```python
from build123d import *

# Parameters (mm, degrees)
F0_W     = 73
F0_H     = 125
F1_DEPTH = 5
F2_D     = 2.5
F3_D     = 3.3
F4_R     = 5
F7_DEPTH = 25
F8_D     = 2.5


# Not quite as in the source:
# - a feature names something its author has since deleted; it is built from what else it names


with BuildPart() as f1:
    # F0 (on Top) → F1 (new body)
    with BuildSketch(Plane.XY):
        with Locations((-1.7126457989, 19.3158909678)):
            Rectangle(F0_W, F0_H)
    extrude(amount=F1_DEPTH)

    # F2 (through all)
    with Locations(Plane(origin=(0, 0, 0), x_dir=(1, 0, 0), z_dir=(0, 0, -1))):
        with Locations((-30.3091388196, -76.7177641392), (27.6908611804, -76.7177641392), (27.6908611804, -53.7177641392), (-30.3091388196, -53.7177641392)):
            Hole(F2_D / 2)

    # F3 (through all)
    with Locations(Plane(origin=(0, 0, 0), x_dir=(1, 0, 0), z_dir=(0, 0, -1))):
        with Locations((-21.0855398327, -47.0293052495), (-13.0855398327, -47.0293052495)):
            Hole(F3_D / 2)

    # F4
    f4_edges = [f1.edges().sort_by_distance(p)[0] for p in [
        (-38.212646, 81.815891, 2.5),
        (34.787354, 81.815891, 2.5),
        (34.787354, -43.184109, 2.5),
        (-38.212646, -43.184109, 2.5),
    ]]
    fillet(f4_edges, radius=F4_R)

    # F5 (on face) → F7 (cut)
    with BuildSketch(Plane.XY.offset(5)):
        Polygon((19.4577450805, 31.105422746), (2.7185706181, 48.1802586667), (-26.0799791984, 20.3202102417), (-26.0799791984, -12.9482956412), align=None)
        Polygon((29.5474557331, 26.9350063375), (-26.0799791984, -26.8796142191), (29.5474557331, -26.8796142191), align=None)
        Polygon((-3.3391041424, 52.5376833975), (23.1605084746, 78.173713526), (-26.1079283048, 78.173713526), (-26.1079283048, 52.5376833975), align=None)
    extrude(amount=-F7_DEPTH, mode=Mode.SUBTRACT)

    # F8 (through all)
    with Locations(Plane.XY.offset(5)):
        with Locations((-29.995566234, 38.7779349625), (18.504433766, 45.4779349625), (18.504433766, -37.4220650375), (-29.995566234, -36.1220650375)):
            Hole(F8_D / 2)


solid = f1.part
```
Read the model definition and answer for the solid it produces. Units are mm, in the model's axes. A direction names the side the tool comes from. Coordinates: 2 decimals unless noted, no trailing zeros. Loops run counter-clockwise (first coordinate to the right, second up) from the corner with the lowest first, then second, coordinate; pieces in that order, holes last. Notation, with made-up numbers: (88.5, 62) - (108.5, 62) arc R22 cw to (108.5, 84) - close; hole circle Ø5 at (-15, 67.25). An arc over 180 degrees is marked (long way). Answer in a Markdown table with one row per item.
1. Find section C-C, the plane y = -25. Write down the section's boundary in (x, z), then the cut area to 3 significant figures.
Conclusion:
| item | result |
|---|---|
| outline | (-38.21, 0) - (-24.14, 0) - (-24.14, 5) - (-38.21, 5) - close; (29.55, 0) - (34.79, 0) - (34.79, 5) - (29.55, 5) - close |
| area | 96.6 mm² |
2. Find section A-A, the plane x = -1. Write down the section's boundary in (y, z), then the cut area to 3 significant figures.
Conclusion:
| item | result |
|---|---|
| outline | (-43.18, 0) - (-26.88, 0) - (-26.88, 5) - (-43.18, 5) - close; (-2.62, 0) - (11.31, 0) - (11.31, 5) - (-2.62, 5) - close; (44.58, 0) - (54.8, 0) - (54.8, 5) - (44.58, 5) - close; (78.17, 0) - (81.82, 0) - (81.82, 5) - (78.17, 5) - close |
| area | 220 mm² |
3. Which of the six approach directions +Z, -Z, +X, -X, +Y, -Y give full straight-line access (tool end or side, diameter ignored) to faces 1 (the face through (2.12, 0.4, 2.54)), 2 (the face through (-36.8, 80.3, 2.5))?
Conclusion:
| item | result |
|---|---|
| face 1 | +Z, -Z |
| face 2 | +Z, -Z, -X, +Y |
4. Straight lines are drawn through the part: line 1 (X direction, y = 17.5, z = 0.6); line 2 (X direction, y = 12.5, z = 2.85); line 3 (Y direction, x = 5, z = 0.2). For each, find the intervals that lie inside material, in ascending order.
Conclusion:
| item | result |
|---|---|
| line 1 | x = -38.21 to -26.08, 5.39 to 19.79, 29.55 to 34.79 |
| line 2 | x = -38.21 to -26.08, 0.23 to 14.63, 29.55 to 34.79 |
| line 3 | y = -43.18 to -26.88, 3.19 to 17.12, 45.85 to 60.61, 78.17 to 81.82 |
5. Find section B-B, the plane y = 9.5. Write down the section's boundary in (x, z), then the cut area to 3 significant figures.
Conclusion:
| item | result |
|---|---|
| outline | (-38.21, 0) - (-26.08, 0) - (-26.08, 5) - (-38.21, 5) - close; (-2.88, 0) - (11.53, 0) - (11.53, 5) - (-2.88, 5) - close; (29.55, 0) - (34.79, 0) - (34.79, 5) - (29.55, 5) - close |
| area | 159 mm² |
6. Determine the mould class of faces 3 (the face through (34.787, 19, 2)), 4 (the face through (-38.213, 19, 2)), 5 (the face through (-2, 81.816, 2)), 6 (the face through (-29.06, 53.66, 2.53)) for opening direction X: +X half, -X half, draft (parallel to the pull), parting line (faces both ways), or undercut.
Conclusion:
| item | result |
|---|---|
| face 3 | +X half |
| face 4 | -X half |
| face 5 | draft |
| face 6 | undercut |
7. Find section D-D, the plane x = -13. Write down the section's boundary in (y, z).
Conclusion:
| item | result |
|---|---|
| outline | (-43.18, 0) - (-26.88, 0) - (-26.88, 5) - (-43.18, 5) - close; (-14.23, 0) - (-0.29, 0) - (-0.29, 5) - (-14.23, 5) - close; (32.97, 0) - (45.38, 0) - (45.38, 5) - (32.97, 5) - close; (48.68, 0) - (52.54, 0) - (52.54, 5) - (48.68, 5) - close; (78.17, 0) - (81.82, 0) - (81.82, 5) - (78.17, 5) - close |
